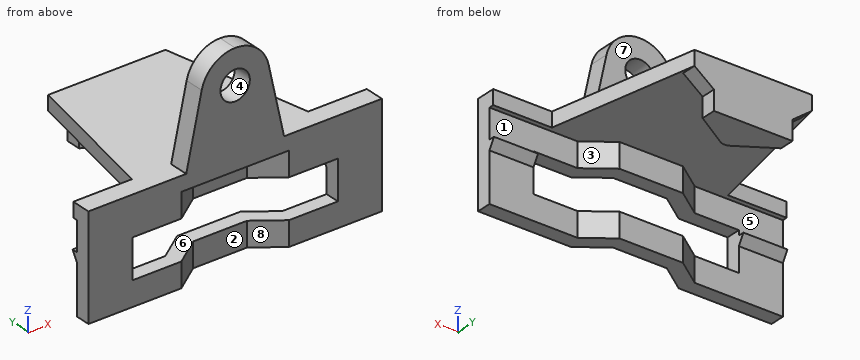
from build123d import *

# Parameters (mm, degrees)
SALIENTE_EXTRUIR1_DEPTH = 1.5
CROQUIS2_W              = 10
CROQUIS2_H              = 2
SALIENTE_EXTRUIR2_DEPTH = 10
CROQUIS3_R              = 1.5
CORTAR_EXTRUIR1_DEPTH   = 10
SALIENTE_EXTRUIR5_DEPTH = 1.5
SALIENTE_EXTRUIR6_DEPTH = 1.5
REDONDEO2_R             = 1
SALIENTE_EXTRUIR7_DEPTH = 9
CORTAR_EXTRUIR2_REACH   = 27.421
CROQUIS8_W              = 21
CROQUIS8_H              = 4
SALIENTE_EXTRUIR8_DEPTH = 4.5
SALIENTE_EXTRUIR9_DEPTH = 4.5


with BuildPart() as part:
    # Croquis1 → Saliente-Extruir1 (new body)
    with BuildSketch(Plane.XY):
        Polygon((-6, 8.5), (6, 8.5), (9, -6.5), (15, -6.5), (15, -8.5), (-15, -8.5), (-15, -6.5), (-9, -6.5), align=None)
    extrude(amount=SALIENTE_EXTRUIR1_DEPTH)

    # Croquis2 → Saliente-Extruir2 (add)
    with BuildSketch(Plane.XY.offset(1.5)):
        with Locations((0, -7.5)):
            Rectangle(CROQUIS2_W, CROQUIS2_H)
    extrude(amount=SALIENTE_EXTRUIR2_DEPTH)

    # Croquis3 → Cortar-Extruir1 (cut)
    with BuildSketch(Plane.XZ.offset(8.5)):
        with BuildLine():
            Line((-5, 11.5), (-5, 1.5))
            Line((-5, 1.5), (-3.41960618, 8.745850907))
            ThreePointArc((-3.41960618, 8.745850907), (-2.195395389, 10.72584649), (0, 11.5))
            Line((0, 11.5), (-5, 11.5))
        make_face()
        with BuildLine():
            Line((5, 11.5), (0, 11.5))
            ThreePointArc((0, 11.5), (2.195395389, 10.72584649), (3.41960618, 8.745850907))
            Line((3.41960618, 8.745850907), (5, 1.5))
            Line((5, 1.5), (5, 11.5))
        make_face()
        with Locations(Location((0, 8, 0), (0, 0, 270))):
            Circle(CROQUIS3_R)
    extrude(amount=-CORTAR_EXTRUIR1_DEPTH, mode=Mode.SUBTRACT)

    # Croquis4 → Saliente-Extruir5 (add)
    with BuildSketch(Plane(origin=(0, 8.5, 0), x_dir=(1, 0, 0), z_dir=(0, 1, 0))):
        Polygon((6, 0), (4.010944544, 1.5), (4.010944544, 3.5), (-4.010944544, 3.5), (-4.010944544, 1.5), (-6, 0), align=None)
    extrude(amount=-SALIENTE_EXTRUIR5_DEPTH)

    # Croquis6 → Saliente-Extruir6 (add)
    with BuildSketch(Plane(origin=(0, 0, -3.5), x_dir=(-1, 0, 0), z_dir=(0, 0, -1))):
        Polygon((-4.010944544, 7), (0, 4.5), (4.010944544, 7), align=None)
    extrude(amount=-SALIENTE_EXTRUIR6_DEPTH)

    # Redondeo2
    redondeo2_edges = [part.edges().sort_by_distance(p)[0] for p in [
        (0, 4.5, -2.75),
    ]]
    fillet(redondeo2_edges, radius=REDONDEO2_R)

    # Croquis7 → Saliente-Extruir7 (add)
    with BuildSketch(Plane(origin=(0, 0, 0), x_dir=(-1, 0, 0), z_dir=(0, 0, -1))):
        Polygon((5.5, -8.5), (15, -8.5), (15, -7), (5.98777572, -7), (3.23777572, -5), (-3.23777572, -5), (-5.98777572, -7), (-15, -7), (-15, -8.5), (-5.5, -8.5), (-2.75, -6.5), (2.75, -6.5), align=None)
    extrude(amount=SALIENTE_EXTRUIR7_DEPTH)

    # Croquis8 → Cortar-Extruir2 (cut, up to next)
    with BuildSketch(Plane.XZ.offset(8.5), mode=Mode.PRIVATE) as cortar_extruir2_sk1:
        with Locations((0, -4.5)):
            Rectangle(CROQUIS8_W, CROQUIS8_H)
    cortar_extruir2_tool1 = extrude(cortar_extruir2_sk1.sketch, amount=-CORTAR_EXTRUIR2_REACH, mode=Mode.PRIVATE) & part.part
    add(cortar_extruir2_tool1.solids().sort_by_distance((0, -8.5, -4.5))[0], mode=Mode.SUBTRACT)

    # Croquis9 → Saliente-Extruir8 (add)
    with BuildSketch(Plane(origin=(15, 0, 0), x_dir=(0, 0, -1), z_dir=(1, 0, 0))):
        Polygon((3, -7), (3, -6.4), (4, -7), align=None)
    extrude(amount=-SALIENTE_EXTRUIR8_DEPTH)

    # Croquis10 → Saliente-Extruir9 (add)
    with BuildSketch(Plane.ZY.offset(15)):
        Polygon((-3, -6.4), (-3, -7), (-4, -7), align=None)
    extrude(amount=-SALIENTE_EXTRUIR9_DEPTH)


solid = part.part
Geometry check sheet. Reference: the model listing, model coordinates, mm. Face numbers are marked on the shaded views. A direction names the side the tool comes from. Round coordinates to 2 decimals unless told otherwise and drop trailing zeros. Loops run counter-clockwise (first coordinate to the right, second up) from the corner with the lowest first, then second, coordinate; pieces in that order, holes last.
Item 1: Mould release check, pull along X, two halves, no side actions. Record for the marked faces 1, 2, 3 and 4: pulls with the +X half, pulls with the -X half, needs draft (parallel to the pull), parting line crosses it, or undercut.
Item 2: Thickness scan on line 1 (Z direction, x = 1.75, y = 6); line 2 (Z direction, x = 4.75, y = 2.5); line 3 (Y direction, x = -0.5, z = -7.5). Record the ranges inside material, lowest first.
Item 3: Gauge pin test, flat ends, axial feed: pin 1 (1.5 mm diameter, centred on x = 10, z = -7, fed in from +Y); pin 2 (3 mm diameter, centred on x = -0.5, z = 6.5, fed in from +Y); pin 3 (4.5 mm diameter, centred on x = 6.5, y = 3, fed in from -Z); pin 4 (8 mm diameter, centred on x = 8, z = -3, fed in from +Y). Record the tip position at first contact, or that the pin passes through.
Item 4: Cross-section at B-B on z = -4.5. Record the boundary of the cut face in (x, y), then the cut area to 3 significant figures.
Item 5: Access from +Z, -Z, +X, -X, +Y, -Y to the whole of each face (thin tool, end or side, straight path). Record for the marked faces 5, 6, 7 and 8.
Item 6: Cross-section at A-A on x = -7. Record the boundary of the cut face in (y, z).
Item 7: Cross-section at C-C on z = -7.5. Record the boundary of the cut face in (x, y), then the cut area to 3 significant figures.
Item 8: Cross-section at D-D on y = -6. Record the boundary of the cut face in (x, z), then the cut area to 3 significant figures.
Answer sheet:
1. face 1: needs draft
1. face 2: undercut
1. face 3: pulls with the +X half
1. face 4: undercut
2. line 1: z = -3.5 to -2, 0 to 1.5
2. line 2: z = 0 to 1.5
2. line 3: y = -6.5 to -5
3. pin 1: stops at y = -7
3. pin 2: stops at y = -6.5
3. pin 3: stops at z = 0
3. pin 4: stops at y = 8.5
4. outline: (-15, -8.5) - (-10.5, -8.5) - (-10.5, -7) - (-15, -7) - close; (10.5, -8.5) - (15, -8.5) - (15, -7) - (10.5, -7) - close
4. area: 13.5 mm2
5. face 5: -X, +Y
5. face 6: +Y, -Y
5. face 7: +Z, +X, -X, +Y
5. face 8: -Z, -Y
6. outline: (-8.5, -9) - (-7, -9) - (-7, -6.5) - (-8.5, -6.5) - close; (-8.5, -2.5) - (-7, -2.5) - (-7, 0) - (3.5, 0) - (3.5, 1.5) - (-8.5, 1.5) - close
7. outline: (-15, -8.5) - (-5.5, -8.5) - (-2.75, -6.5) - (2.75, -6.5) - (5.5, -8.5) - (15, -8.5) - (15, -7) - (5.99, -7) - (3.24, -5) - (-3.24, -5) - (-5.99, -7) - (-15, -7) - close
7. area: 47.0 mm2
8. outline: (-8.9, 0) - (-4.61, 0) - (-4.61, -2.5) - (4.61, -2.5) - (4.61, 0) - (8.9, 0) - (8.9, 1.5) - (-8.9, 1.5) - close; (-4.61, -9) - (4.61, -9) - (4.61, -6.5) - (-4.61, -6.5) - close
8. area: 72.8 mm2
